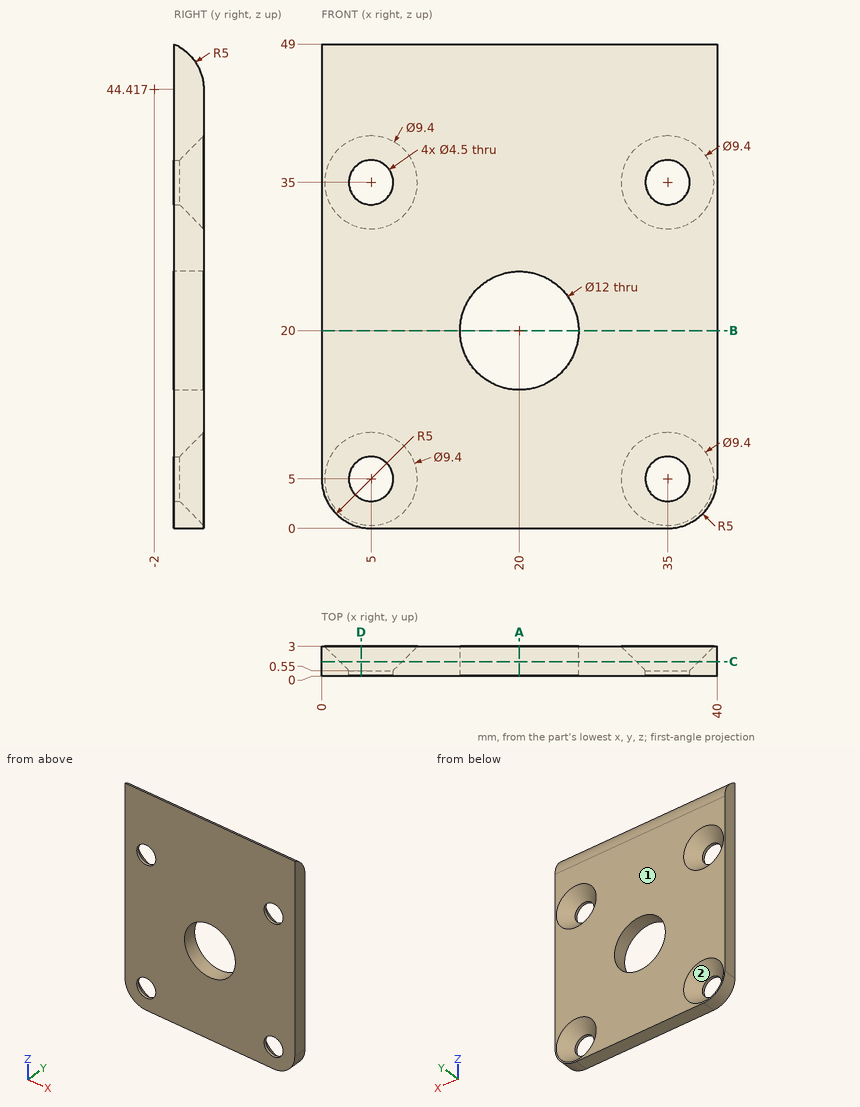
Design review of the part shown in the three views and the two pictorial views. Dimensions are in mm from the part's minimum x, y and z. Round coordinates to 2 decimals unless told otherwise and drop trailing zeros. Loops run counter-clockwise (first coordinate to the right, second up) from the corner with the lowest first, then second, coordinate; pieces in that order, holes last.
Q1. Add section A-A on x = 20. Write out the cut boundary in (y, z).
Result sheet:
outline: (0, 0) - (3, 0) - (3, 14) - (0, 14) - close; (0, 26) - (3, 26) - (3, 44.42) arc R5 ccw to (0, 49) - close
Q2. Insertion check: pin 1 Ø2.5 at (x, z) = (35, 5) entering from +Y; pin 2 Ø1 at (y, z) = (2.5, 12) entering from -X. Each pin has a flat end and moves straight along its axis. Give the tip position at first contact, or say it passes through.
Result sheet:
pin 1: passes through
pin 2: stops at x = 0
Q3. To check wall thickness, follow line 1 along X through (y, z) = (0.45, 35); line 2 along Z through (x, y) = (37, 1.4) (1 decimal); line 3 along Z through (x, y) = (5, 0.3). State the ranges of each line that lie inside material, in increasing order.
Result sheet:
line 1: x = 0 to 2.75, 7.25 to 32.75, 37.25 to 40
line 2: z = 0.4 to 2.6, 7.4 to 32.6, 37.4 to 48.1
line 3: z = 0 to 2.75, 7.25 to 32.75, 37.25 to 48.86
Q4. Add section D-D on x = 4. Give the number of separate pieces and of enclosed holes in the cut face, plus the area to 3 significant figures.
Result sheet:
separate pieces: 3
enclosed holes: 0
area: 106 mm2
Q5. Add section C-C on y = 1.45. Write out the cut boundary in (x, z).
Result sheet:
outline: (0, 5) arc R5 ccw to (5, 0) - (35, 0) arc R5 ccw to (40, 5) - (40, 48.04) - (0, 48.04) - close; hole circle Ø6.3 at (5, 5); hole circle Ø6.3 at (5, 35); hole circle Ø12 at (20, 20); hole circle Ø6.3 at (35, 5); hole circle Ø6.3 at (35, 35)
Q6. Add section B-B on z = 20. Write out the cut boundary in (x, y).
Result sheet:
outline: (0, 0) - (14, 0) - (14, 3) - (0, 3) - close; (26, 0) - (40, 0) - (40, 3) - (26, 3) - close
Q7. Mouldability with a two-part tool opening along X and no side actions: class the marked faces 1 and 2 as +X half, -X half, draft (parallel to the pull), parting line (faces both ways), or undercut.
Result sheet:
face 1: draft
face 2: undercut
